Here's how the part is built. I have some questions about the finished solid (model axes, mm). A direction names the side the tool comes from. Coordinates: 2 decimals unless noted, no trailing zeros. Order: outer loops, then holes, each group sorted by start corner. A loop starts at its lowest first (then second) coordinate and runs counter-clockwise, first axis right, second up. Notation, with made-up numbers: (0, -31) -> (8, -31) arc R32 ccw to (8, 7) -> close; hole circle Ø5 at (44, 30.5). An arc over 180 degrees is marked (long way). One line per item, written item: value. Start each with the question number.
Autodesk Inventor part; units mm, degrees
ref_plane "YZ Plane" through (0, 0, 0) normal (1, 0, 0) x (0, 1, 0)
ref_plane "XZ Plane" through (0, 0, 0) normal (0, 1, 0) x (-1, 0, 0)
ref_plane "XY Plane" through (0, 0, 0) normal (0, 0, 1) x (1, 0, 0)
sketch "Sketch1" plane through (0, 0, 0) normal (0, 1, 0) x (-1, 0, 0)
  line L0 (0, 0) -> (127, 0)
  line L1 (127, 0) -> (127, -651.51)
  line L2 (127, -651.51) -> (0, -651.51)
  line L3 (0, -651.51) -> (0, 0)
  line L4 (123.825, -3.175) -> (3.175, -3.175)
  line L5 (3.175, -3.175) -> (3.175, -648.335)
  line L6 (3.175, -648.335) -> (123.825, -648.335)
  line L7 (123.825, -648.335) -> (123.825, -3.175)
  circle A0 centre (101.6, -478.155) radius 2.3812
  circle A1 centre (25.4, -478.155) radius 2.3813
  line L8 (3.175, -325.755) -> (14.531, -325.755)
  circle A2 centre (101.6, -173.355) radius 2.3812
  circle A3 centre (25.4, -173.355) radius 2.3813
  dimension "d0" = 127
  dimension "d1" = 651.51
  dimension "d2" = 3.175
  dimension "d13" = 4.7625
  dimension "d14" = 4.7625
  dimension "d15" = 76.2
  dimension "d16" = 25.4
  dimension "d17" = 152.4
extrude "Extrusion1" add sketch "Sketch1" along normal blind 3.175 contours L7 L6 L5 L4
extrude "Extrusion2" add sketch "Sketch1" along normal blind 144.78 contours L0 L1 L2 L3
sketch "Sketch2" plane through (0, 0, 0) normal (0, -1, 0) x (1, 0, 0)
  line L0 (-50.8, -76.2) -> (-76.2, -76.2)
  line L1 (-76.2, -76.2) -> (-76.2, -88.9)
  line L2 (-76.2, -88.9) -> (-50.8, -88.9)
  line L3 (-50.8, -88.9) -> (-50.8, -76.2)
  line L4 (0, 0) -> (0, -651.51)
  line L5 (0, -325.755) -> (-127, -325.755)
  line L6 (-127, -651.51) -> (-127, 0)
  line L7 (-50.8, -575.31) -> (-76.2, -575.31)
  line L8 (-76.2, -575.31) -> (-76.2, -562.61)
  line L9 (-76.2, -562.61) -> (-50.8, -562.61)
  line L10 (-50.8, -562.61) -> (-50.8, -575.31)
  line L11 (-127, 0) -> (0, 0)
  dimension "d7" = 25.4
  dimension "d8" = 12.7
  dimension "d9" = 50.8
  dimension "d10" = 76.2
extrude "Extrusion3" add sketch "Sketch2" along normal blind 12.7 contours L3 L2 L1 L0 | L7 L8 L9 L10
extrude "Extrusion4" add sketch "Sketch1" along normal blind 76.2 contours A0 | A1 | A2 | A3
sketch "Sketch3" plane through (0, 3.175, 0) normal (0, 1, 0) x (1, 0, 0)
  line L0 (-3.175, 3.175) -> (-3.175, 648.335)
  line L1 (-123.825, 648.335) -> (-123.825, 3.175)
  line L2 (-3.175, 66.675) -> (-123.825, 66.675)
  line L3 (-123.825, 66.675) -> (-123.825, 117.475)
  line L4 (-123.825, 117.475) -> (-3.175, 117.475)
  line L5 (-3.175, 117.475) -> (-3.175, 66.675)
  line L6 (-3.175, 3.175) -> (-123.825, 3.175)
  line L7 (-127, 651.51) -> (-127, 0)
  line L8 (-127, 325.755) -> (-116.0264, 325.755)
  line L9 (-3.175, 584.835) -> (-123.825, 584.835)
  line L10 (-123.825, 584.835) -> (-123.825, 534.035)
  line L11 (-123.825, 534.035) -> (-3.175, 534.035)
  line L12 (-3.175, 534.035) -> (-3.175, 584.835)
  point P0 (0, 0)
  point P1 (-3.175, 534.035)
  point P2 (-3.175, 117.475)
  dimension "d20" = 50.8
  dimension "d21" = 63.5
extrude "Extrusion5" add sketch "Sketch3" along normal blind 19.05 contours L2 L1 L4 L0 | L11 L1 L9 L0
properties part number "Box"
Q1. Imagine slicing it at C-C (x = -64). Write out the boundary of the cut face in (y, z) (3 decimals).
Q2. I need wall thicknesses on line 1 (Z direction, x = -66, y = 4.5) (3 decimals); line 2 (Z direction, x = -65.5, y = -4.5); line 3 (Z direction, x = -100, y = 60) (3 decimals). Which ranges of each line are inside material? Lowest first, please.
Q3. Imagine slicing it at A-A (y = 9.5). Write out the boundary of the cut face in (x, z) (3 decimals), plus the area to 3 significant figures.
Q4. If we mould it in two halves opening along Z, with no side actions, what happens to faces 6 (the face through (-63, -6, -575.31)), 7 (the face through (-127, 71, -321)), 8 (the face through (-63, 3.175, -616))? For each: +Z half, -Z half, draft (parallel to the pull), parting line (faces both ways), or undercut.
Q5. For faces 1 (the face through (-64, -6, -88.9)), 2 (the face through (-76.2, -6, -82)), 3 (the face through (-50.8, -6, -569)), 4 (the face through (-63, -6, -76.2)), 5 (the face through (-64, 73, -3.175)), which set-ups out of +Z, -Z, +X, -X, +Y, -Y let a thin tool reach every point of the face, with its end or its side?
Q6. For P1, Ø6.5, axis at x = -63, y = -4.5, coming from the -Z side; P2, Ø4, axis at x = -60, y = -5, coming from the +Z side; P3, Ø1, axis at x = -94.5, z = -499.5, coming from the -Y side, each with a flat end and sliding along its axis, tell me the tip position at first contact or that it passes through.
Q7. Imagine slicing it at D-D (y = 46.5). Write out the boundary of the cut face in (x, z) (3 decimals), plus the area to 3 significant figures.
Q8. Imagine slicing it at B-B (z = -457.5). Write out the boundary of the cut face in (x, y) (3 decimals), plus the area to 3 significant figures.
Completed:
1. outline: (-12.7, -575.31) -> (0, -575.31) -> (0, -651.51) -> (144.78, -651.51) -> (144.78, -648.335) -> (3.175, -648.335) -> (3.175, -584.835) -> (22.225, -584.835) -> (22.225, -534.035) -> (3.175, -534.035) -> (3.175, -117.475) -> (22.225, -117.475) -> (22.225, -66.675) -> (3.175, -66.675) -> (3.175, -3.175) -> (144.78, -3.175) -> (144.78, 0) -> (0, 0) -> (0, -76.2) -> (-12.7, -76.2) -> (-12.7, -88.9) -> (0, -88.9) -> (0, -562.61) -> (-12.7, -562.61) -> close
2. line 1: z = -651.51 to -648.335, -584.835 to -534.035, -117.475 to -66.675, -3.175 to 0
2. line 2: z = -575.31 to -562.61, -88.9 to -76.2
2. line 3: z = -651.51 to -648.335, -479.919 to -476.391, -175.119 to -171.591, -3.175 to 0
3. outline: (-127, -651.51) -> (0, -651.51) -> (0, 0) -> (-127, 0) -> close; circle Ø4.762 at (-101.6, -478.155); circle Ø4.762 at (-101.6, -173.355); circle Ø4.763 at (-25.4, -478.155); circle Ø4.763 at (-25.4, -173.355); hole (-123.825, -648.335) -> (-3.175, -648.335) -> (-3.175, -584.835) -> (-123.825, -584.835) -> close; hole (-123.825, -534.035) -> (-3.175, -534.035) -> (-3.175, -117.475) -> (-123.825, -117.475) -> close; hole (-123.825, -66.675) -> (-3.175, -66.675) -> (-3.175, -3.175) -> (-123.825, -3.175) -> close
3. area: 17,200 mm2
4. face 6: -Z half
4. face 7: draft
4. face 8: undercut
5. face 1: +X, -X, -Y
5. face 2: +Z, -Z, -X, -Y
5. face 3: +Z, -Z, +X, -Y
5. face 4: +Z, +X, -X, -Y
5. face 5: +Y
6. P1: stops at z = -575.31
6. P2: stops at z = -76.2
6. P3: stops at y = 0
7. outline: (-127, -651.51) -> (0, -651.51) -> (0, 0) -> (-127, 0) -> close; circle Ø4.762 at (-101.6, -478.155); circle Ø4.762 at (-101.6, -173.355); circle Ø4.763 at (-25.4, -478.155); circle Ø4.763 at (-25.4, -173.355); hole (-123.825, -648.335) -> (-3.175, -648.335) -> (-3.175, -3.175) -> (-123.825, -3.175) -> close
7. area: 4,970 mm2
8. outline: (-127, 0) -> (0, 0) -> (0, 144.78) -> (-3.175, 144.78) -> (-3.175, 3.175) -> (-123.825, 3.175) -> (-123.825, 144.78) -> (-127, 144.78) -> close
8. area: 1,300 mm2
